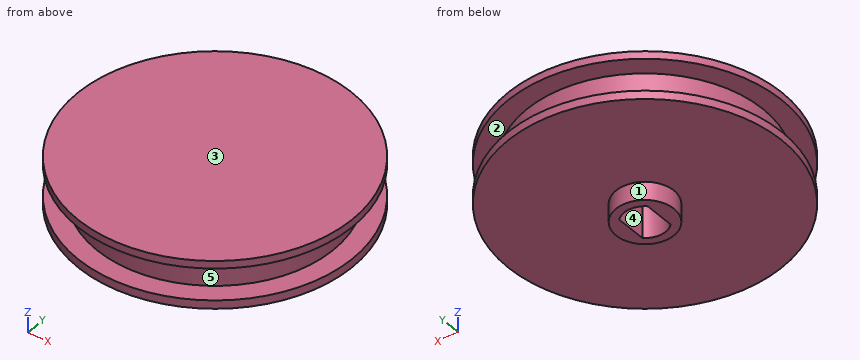
Autodesk Inventor part; units mm, degrees
ref_plane "YZ Plane" through (0, 0, 0) normal (1, 0, 0) x (0, 1, 0)
ref_plane "XZ Plane" through (0, 0, 0) normal (0, 1, 0) x (-1, 0, 0)
ref_plane "XY Plane" through (0, 0, 0) normal (0, 0, 1) x (1, 0, 0)
sketch "Sketch1" plane through (0, 0, 0) normal (0, 0, 1) x (1, 0, 0)
  circle A0 centre (0, 0) radius 4.826
  dimension "d0" = 9.652
extrude "Extrusion1" add sketch "Sketch1" along normal blind 3.048
sketch "Sketch2" plane through (0, 0, 3.048) normal (0, 0, 1) x (1, 0, 0)
  circle A0 centre (0, 0) radius 22.86
  dimension "d3" = 45.72
extrude "Extrusion2" add sketch "Sketch2" along normal blind 1.397
sketch "Sketch4" plane through (0, 0, 4.445) normal (0, 0, 1) x (1, 0, 0)
  circle A0 centre (0, 0) radius 19.685
  dimension "d6" = 39.37
extrude "Extrusion3" add sketch "Sketch4" along normal blind 5.334
sketch "Sketch6" plane through (0, 0, 9.779) normal (0, 0, 1) x (1, 0, 0)
  circle A0 centre (0, 0) radius 4.826
  circle A1 centre (0, 0) radius 22.86
extrude "Extrusion4" add sketch "Sketch6" along normal blind 1.27 contours A0 | A1
sketch "Sketch9" plane through (0, 0, 0) normal (0, 0, -1) x (-1, 0, 0)
  line L0 (2.3876, -2.514) -> (2.3876, 2.514)
  line L1 (-2.3876, 2.514) -> (-2.3876, -2.514)
  line L2 (-1.2735, -3.2247) -> (1.2735, 3.2247) construction
  line L3 (1.2735, -3.2247) -> (-1.2735, 3.2247) construction
  arc A0 (-2.3876, -2.514) -> (2.3876, -2.514) centre (0, 0) ccw
  arc A1 (2.3876, 2.514) -> (-2.3876, 2.514) centre (0, 0) ccw
extrude "Extrusion6" cut sketch "Sketch9" against normal blind 5.5118
properties part number "Wheel"
Part model, mm, in its own coordinate system. Face numbers are marked on the shaded views. A direction names the side the tool comes from. Round coordinates to 2 decimals unless told otherwise and drop trailing zeros. Order: outer loops, then holes, each group sorted by start corner. A loop starts at its lowest first (then second) coordinate and runs counter-clockwise, first axis right, second up. Notation, with made-up numbers: M 60.25,-8.5 L 118.25,-8.5 A33 ccw 118.25,21.5 Z; hole C 31.25,15 d5. An arc over 180 degrees is marked long. Answer in a Markdown table with one row per item. Add a question column.
Q1. 3-axis set-ups, long thin cutter, end or side, ignore diameter. For the marked faces 4 and 5: which of +Z, -Z, +X, -X, +Y, -Y reach the whole face in a straight line?
Q2. Pin check, flat tips, straight feed: pin 1 (5.5 mm diameter, centred on y = 0, z = 3, fed in from +X); pin 2 (3 mm diameter, centred on y = 9, z = 9, fed in from +X); pin 3 (1 mm diameter, centred on y = -8.5, z = 6.5, fed in from -X); pin 4 (6 mm diameter, centred on x = 6, z = 1.5, fed in from +Y). Stop position of each tip, or through.
Q3. Cut at A-A on z = 2. Give the cut face in (x, y), and give its area (3 significant figures).
Q4. Cut at B-B on y = 0. Give the cut face in (x, z) (3 decimals).
Q5. Wall check: L1, parallel to Z at x = 19, y = -6 (3 decimals); L2, parallel to Z at x = 2, y = -12.5; L3, parallel to X at y = -6, z = 4.5. Give the ranges that are in metal, low to high. Write a range as from..to.
Q6. Mould opens along Z. For the marked faces 1, 2 and 3 say: +Z half, -Z half, draft (parallel to the pull), parting line (faces both ways), or undercut.
Q7. Cut at D-D on z = 7.75. Give the cut face in (x, y) (3 decimals).
Q8. Cut at C-C on x = 0. Give the cut face in (y, z) (3 decimals), and give its area (3 significant figures).
Established:
| question | item | result |
|---|---|---|
| 1 | face 4 | -Z |
| 1 | face 5 | none |
| 2 | pin 1 | stops at x = 22.86 |
| 2 | pin 2 | stops at x = 21.52 |
| 2 | pin 3 | stops at x = -17.99 |
| 2 | pin 4 | stops at y = 22.6 |
| 3 | outline | C 0,0 d9.65; hole M -2.39,-2.51 A3.47 ccw 2.39,-2.51 L 2.39,2.51 A3.47 ccw -2.39,2.51 Z |
| 3 | area | 42.9 mm2 |
| 4 | outline | M -22.86,3.048 L -4.826,3.048 L -4.826,0 L -2.388,0 L -2.388,5.512 L 2.388,5.512 L 2.388,0 L 4.826,0 L 4.826,3.048 L 22.86,3.048 L 22.86,4.445 L 19.685,4.445 L 19.685,9.779 L 22.86,9.779 L 22.86,11.049 L -22.86,11.049 L -22.86,9.779 L -19.685,9.779 L -19.685,4.445 L -22.86,4.445 Z |
| 5 | L1 | z = 3.048..4.445, 9.779..11.049 |
| 5 | L2 | z = 3.05..11.05 |
| 5 | L3 | x = -18.75..18.75 |
| 6 | face 1 | draft |
| 6 | face 2 | undercut |
| 6 | face 3 | +Z half |
| 7 | outline | C 0,0 d39.37 |
| 8 | outline | M -22.86,3.048 L -4.826,3.048 L -4.826,0 L -3.467,0 L -3.467,5.512 L 3.467,5.512 L 3.467,0 L 4.826,0 L 4.826,3.048 L 22.86,3.048 L 22.86,4.445 L 19.685,4.445 L 19.685,9.779 L 22.86,9.779 L 22.86,11.049 L -22.86,11.049 L -22.86,9.779 L -19.685,9.779 L -19.685,4.445 L -22.86,4.445 Z |
| 8 | area | 323 mm2 |
